```python
from build123d import *

# Parameters (mm, degrees)
SKETCH1_W           = 10
SKETCH1_H           = 15
SKETCH1_R           = 4.95
SKETCH1_R_2         = 2.5
BOSS_EXTRUDE1_DEPTH = 3
BOSS_EXTRUDE2_START = -3
SKETCH1_3_W         = 10
SKETCH1_3_H         = 15
SKETCH1_3_R         = 4.95
SKETCH1_3_R_2       = 2.5
BOSS_EXTRUDE2_DEPTH = 3
CUT_EXTRUDE1_START  = 1.5
SKETCH1_4_R         = 4.95
SKETCH1_4_R_2       = 2.5
CUT_EXTRUDE1_DEPTH  = 1.5


with BuildPart() as part:
    # Sketch1 → Boss-Extrude1 (new body)
    # profile 1 of 6: a face of its own
    with BuildSketch(Plane.XY):
        with Locations((-37.532834977, 11.935892272)):
            Rectangle(SKETCH1_W, SKETCH1_H)
        with Locations((-37.532834977, 9.435892272)):
            Circle(SKETCH1_R, mode=Mode.SUBTRACT)
    # profile 2 of 6: a face of its own
    with BuildSketch(Plane.XY):
        with Locations((-37.532834977, 9.435892272)):
            Circle(SKETCH1_R)
        with Locations((-37.532834977, 9.435892272)):
            Circle(SKETCH1_R_2, mode=Mode.SUBTRACT)
    # profile 3 of 6: a face of its own
    with BuildSketch(Plane.XY):
        with Locations((-7.532834977, 11.935892272)):
            Rectangle(SKETCH1_W, SKETCH1_H)
        with Locations((-7.532834977, 9.435892272)):
            Circle(SKETCH1_R, mode=Mode.SUBTRACT)
    # profile 4 of 6: a face of its own
    with BuildSketch(Plane.XY):
        with Locations((-7.532834977, 9.435892272)):
            Circle(SKETCH1_R)
        with Locations((-7.532834977, 9.435892272)):
            Circle(SKETCH1_R_2, mode=Mode.SUBTRACT)
    # profile 5 of 6: a face of its own
    with BuildSketch(Plane.XY):
        with Locations((-17.532834977, 11.935892272)):
            Rectangle(SKETCH1_W, SKETCH1_H)
    # profile 6 of 6: a face of its own
    with BuildSketch(Plane.XY):
        with Locations((-27.532834977, 11.935892272)):
            Rectangle(SKETCH1_W, SKETCH1_H)
    extrude(amount=BOSS_EXTRUDE1_DEPTH)

    # Sketch1<3> → Boss-Extrude2 (add)
    # profile 1 of 4: a face of its own
    with BuildSketch(Plane.XY.offset(BOSS_EXTRUDE2_START)):
        with Locations((-37.532834977, 11.935892272)):
            Rectangle(SKETCH1_3_W, SKETCH1_3_H)
        with Locations((-37.532834977, 9.435892272)):
            Circle(SKETCH1_3_R, mode=Mode.SUBTRACT)
    # profile 2 of 4: a face of its own
    with BuildSketch(Plane.XY.offset(BOSS_EXTRUDE2_START)):
        with Locations((-37.532834977, 9.435892272)):
            Circle(SKETCH1_3_R)
        with Locations((-37.532834977, 9.435892272)):
            Circle(SKETCH1_3_R_2, mode=Mode.SUBTRACT)
    # profile 3 of 4: a face of its own
    with BuildSketch(Plane.XY.offset(BOSS_EXTRUDE2_START)):
        with Locations((-7.532834977, 11.935892272)):
            Rectangle(SKETCH1_3_W, SKETCH1_3_H)
        with Locations((-7.532834977, 9.435892272)):
            Circle(SKETCH1_3_R, mode=Mode.SUBTRACT)
    # profile 4 of 4: a face of its own
    with BuildSketch(Plane.XY.offset(BOSS_EXTRUDE2_START)):
        with Locations((-7.532834977, 9.435892272)):
            Circle(SKETCH1_3_R)
        with Locations((-7.532834977, 9.435892272)):
            Circle(SKETCH1_3_R_2, mode=Mode.SUBTRACT)
    extrude(amount=BOSS_EXTRUDE2_DEPTH)

    # Sketch1<4> → Cut-Extrude1 (cut)
    # profile 1 of 2: a face of its own
    with BuildSketch(Plane.XY.offset(CUT_EXTRUDE1_START)):
        with Locations((-37.532834977, 9.435892272)):
            Circle(SKETCH1_4_R)
        with Locations((-37.532834977, 9.435892272)):
            Circle(SKETCH1_4_R_2, mode=Mode.SUBTRACT)
    # profile 2 of 2: a face of its own
    with BuildSketch(Plane.XY.offset(CUT_EXTRUDE1_START)):
        with Locations((-7.532834977, 9.435892272)):
            Circle(SKETCH1_4_R)
        with Locations((-7.532834977, 9.435892272)):
            Circle(SKETCH1_4_R_2, mode=Mode.SUBTRACT)
    extrude(amount=CUT_EXTRUDE1_DEPTH, mode=Mode.SUBTRACT)


solid = part.part
```
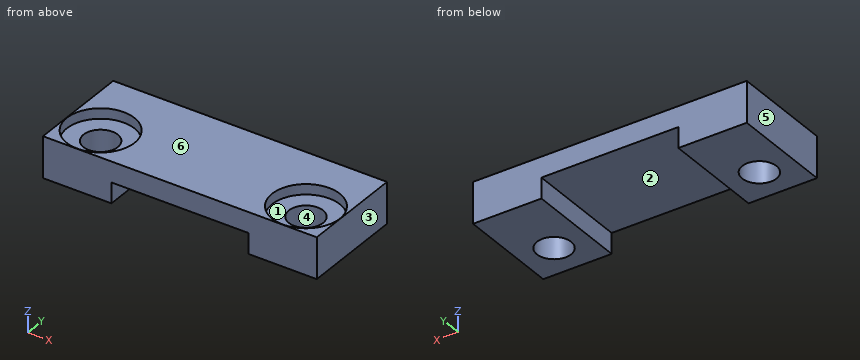
Source: CAD feature listing. Evaluate the final solid. Frame: model axes, mm. Face numbers are marked on the shaded views. A direction names the side the tool comes from. Round coordinates to 2 decimals unless told otherwise and drop trailing zeros. Loops run counter-clockwise (first coordinate to the right, second up) from the corner with the lowest first, then second, coordinate; pieces in that order, holes last. Notation, with made-up numbers: (22.25, 14) - (47.25, 14) arc R20 ccw to (47.25, 34) - close; hole circle Ø8 at (52, 0). An arc over 180 degrees is marked (long way). Use CSV: the item, a comma, the result in double quotes.
Q1. Ray query, line 1 along X through (y, z) = (13, -1.75); line 2 along X through (y, z) = (8, -1.5); line 3 along X through (y, z) = (9, -2.7). Return the intervals inside material, ascending.
Reported:
line 1,"-42.53 to -32.53, -12.53 to -2.53"
line 2,"-42.53 to -39.58, -35.49 to -32.53, -12.53 to -9.58, -5.49 to -2.53"
line 3,"-42.53 to -39.99, -35.07 to -32.53, -12.53 to -9.99, -5.07 to -2.53"
Q2. Pin query (flat end, axial travel): pin 1 Ø5 at (x, y) = (-8, 11) entering from +Z; pin 2 Ø1 at (x, z) = (-13.5, -1) entering from +Y; pin 3 Ø7.5 at (x, y) = (-23, 15.5) entering from -Z. Return the tip coordinate at first contact, or that it passes through.
Reported:
pin 1,"z = 1.5"
pin 2,"through"
pin 3,"z = 0"
Q3. Mould query, pull axis X, two halves, no side actions, for the marked faces 4, 5 and 6. Classes: pulls with the +X half, pulls with the -X half, needs draft (parallel to the pull), parting line crosses it, or undercut.
Reported:
face 4,"undercut"
face 5,"pulls with the -X half"
face 6,"needs draft"
Q4. Section query A-A, the plane z = -1.5. Output: boundary loops of the cut face in (x, y), then the cut area to 3 significant figures.
Reported:
outline,"(-42.53, 4.44) - (-32.53, 4.44) - (-32.53, 19.44) - (-42.53, 19.44) - close; (-12.53, 4.44) - (-2.53, 4.44) - (-2.53, 19.44) - (-12.53, 19.44) - close; hole circle Ø5 at (-37.53, 9.44); hole circle Ø5 at (-7.53, 9.44)"
area,"261 mm^2"
Q5. Section query C-C, the plane y = 10.25. Output: boundary loops of the cut face in (x, z), then the cut area to 3 significant figures.
Reported:
outline,"(-42.53, -3) - (-39.9, -3) - (-39.9, 1.5) - (-42.42, 1.5) - (-42.42, 3) - (-42.53, 3) - close; (-35.17, -3) - (-32.53, -3) - (-32.53, 0) - (-12.53, 0) - (-12.53, -3) - (-9.9, -3) - (-9.9, 1.5) - (-12.42, 1.5) - (-12.42, 3) - (-32.65, 3) - (-32.65, 1.5) - (-35.17, 1.5) - close; (-5.17, -3) - (-2.53, -3) - (-2.53, 3) - (-2.65, 3) - (-2.65, 1.5) - (-5.17, 1.5) - close"
area,"108 mm^2"
Q6. Section query D-D, the plane y = 15.5. Output: boundary loops of the cut face in (x, z).
Reported:
outline,"(-42.53, -3) - (-32.53, -3) - (-32.53, 0) - (-12.53, 0) - (-12.53, -3) - (-2.53, -3) - (-2.53, 3) - (-42.53, 3) - close"
Q7. Section query B-B, the plane x = -37.5. Output: boundary loops of the cut face in (y, z), then the cut area to 3 significant figures.
Reported:
outline,"(4.44, -3) - (6.94, -3) - (6.94, 1.5) - (4.49, 1.5) - (4.49, 3) - (4.44, 3) - close; (11.94, -3) - (19.44, -3) - (19.44, 3) - (14.39, 3) - (14.39, 1.5) - (11.94, 1.5) - close"
area,"52.7 mm^2"
Q8. Reachability of the marked faces 1, 2 and 3 from +Z, -Z, +X, -X, +Y, -Y: full face, straight path, thin tool, end or side. Return the list, or none.
Reported:
face 1,"+Z"
face 2,"-Z, +Y, -Y"
face 3,"+Z, -Z, +X, +Y, -Y"
